Build history of the part. All positions in model axes, mm. A direction names the side the tool comes from. Round coordinates to 2 decimals unless told otherwise and drop trailing zeros. Loops run counter-clockwise (first coordinate to the right, second up) from the corner with the lowest first, then second, coordinate; pieces in that order, holes last. Notation, with made-up numbers: (-25, -9.75) - (-10, -9.75) arc R21 cw to (-10, 29.25) - close; hole circle Ø8 at (-4.75, 33.5). An arc over 180 degrees is marked (long way). Use a Markdown table: item, result.
from build123d import *

# Parameters (mm, degrees)
F0_R     = 48.895
F0_R_2   = 1.5875
F1_DEPTH = 9.525
F0_R_3   = 50.8
F2_DEPTH = 9.525
F3_DEPTH = 1.27


with BuildPart() as f1:
    # F0 (on Front) → F1 (new body, symmetric)
    with BuildSketch(Plane.XZ):
        with Locations((-23.888467, 6.381166)):
            Circle(F0_R)
        with Locations((-23.888467, 6.381166)):
            Circle(F0_R_2, mode=Mode.SUBTRACT)
    extrude(amount=F1_DEPTH, both=True)

    # F0 (on Front) → F2 (join, symmetric)
    with BuildSketch(Plane.XZ):
        with Locations((-23.888467, 6.381166)):
            Circle(F0_R_3)
        with Locations((-23.888467, 6.381166)):
            Circle(F0_R, mode=Mode.SUBTRACT)
    extrude(amount=F2_DEPTH, both=True)

    # F0 (on Front) → F3 (cut, symmetric)
    with BuildSketch(Plane.XZ):
        with Locations((-23.888467, 6.381166)):
            Circle(F0_R_3)
        with Locations((-23.888467, 6.381166)):
            Circle(F0_R, mode=Mode.SUBTRACT)
    extrude(amount=F3_DEPTH, both=True, mode=Mode.SUBTRACT)


solid = f1.part
Q1. Which spindle directions (+Z, -Z, +X, -X, +Y, -Y) get a long thin tool onto all of the face, cutting with end or side? Do faces 1 (the face through (-25, -9.525, -4)), 2 (the face through (-50, -1.27, 48)). Say none if no direction does.
Results found:
| item | result |
|---|---|
| face 1 | +Z, -Z, +X, -X, -Y |
| face 2 | none |
Q2. Drop flat-ended pins along their axis: pin 1 (4 mm diameter, centred on y = -7, z = -29, fed in from +X); pin 2 (3 mm diameter, centred on x = -41, y = -3.5, fed in from -Z); pin 3 (8 mm diameter, centred on y = 4.5, z = -6, fed in from -X). Give the stop position or say it passes through.
Results found:
| item | result |
|---|---|
| pin 1 | stops at x = 14.4 |
| pin 2 | stops at z = -41.96 |
| pin 3 | stops at x = -73.99 |
Q3. Pull direction X, two halves, no side cores. Call faces 3 (the face through (-25, 9.525, -4)), 4 (the face through (22.75, 0.02, 21.07)), 5 (the face through (-22.422, 0.133, 5.773)): pulls with the +X half, pulls with the -X half, needs draft (parallel to the pull), parting line crosses it, or undercut.
Results found:
| item | result |
|---|---|
| face 3 | needs draft |
| face 4 | parting line crosses it |
| face 5 | undercut |
Q4. Probe line 1 (Z direction, x = -5, y = 1.5); line 2 (Z direction, x = -64.5, y = 1); line 3 (X direction, y = 6.5, z = -16.5). List the from-to ranges inside material, lowest first.
Results found:
| item | result |
|---|---|
| line 1 | z = -40.78 to 53.54 |
| line 2 | z = -20.85 to 33.61 |
| line 3 | x = -69.24 to 21.47 |
Q5. Cut at A-A, the plane z = -35. List the corners of the cut face in (x, y) (3 decimals).
Results found:
| item | result |
|---|---|
| outline | (-53.354, -9.525) - (5.577, -9.525) - (5.577, -1.27) - (2.156, -1.27) - (2.156, 1.27) - (5.577, 1.27) - (5.577, 9.525) - (-53.354, 9.525) - (-53.354, 1.27) - (-49.933, 1.27) - (-49.933, -1.27) - (-53.354, -1.27) - close |
Q6. Cut at C-C, the plane y = 4.75. List the corners of the cut face in (x, z) (1 decimal).
Results found:
| item | result |
|---|---|
| outline | circle Ø101.6 at (-23.9, 6.4); hole circle Ø3.2 at (-23.9, 6.4) |
Q7. Cut at B-B, the plane x = -10. List the corners of the cut face in (y, z) (3 decimals), plus the area to 3 significant figures.
Results found:
| item | result |
|---|---|
| outline | (-9.525, -42.483) - (-1.27, -42.483) - (-1.27, -40.5) - (1.27, -40.5) - (1.27, -42.483) - (9.525, -42.483) - (9.525, 55.246) - (1.27, 55.246) - (1.27, 53.262) - (-1.27, 53.262) - (-1.27, 55.246) - (-9.525, 55.246) - close |
| area | 1,850 mm2 |
